Input: dimensioned drawing with shaded views. Units: mm. Origin: part minimum x, y, z. A direction names the side the tool comes from. Coordinates: 2 decimals unless noted, no trailing zeros. Loops run counter-clockwise (first coordinate to the right, second up) from the corner with the lowest first, then second, coordinate; pieces in that order, holes last.
Item 1: Line query: probe 1 along X at (y, z) = (4.75, 2.75); probe 2 along Z at (x, y) = (40, 4); probe 3 along X at (y, z) = (14.5, 25). Output: solid intervals per line, ascending.
Item 2: Section query D-D, the plane z = 27.75. Return the cut outline in (x, y), then the cut area to 3 significant figures.
Item 3: Reachability of the marked faces 1, 2 and 3 from +Z, -Z, +X, -X, +Y, -Y: full face, straight path, thin tool, end or side. Return the list, or none.
Item 4: Pull-direction query (Z, two-part tool) for the marked faces 4, 5, 6 and 7; classes: +Z half, -Z half, draft (parallel to the pull), parting line (faces both ways), or undercut.
Item 5: Section query B-B, the plane y = 10. Return the cut outline in (x, z), then the cut area to 3 significant figures.
Item 6: Section query A-A, the plane z = 8.75. Return the cut outline in (x, y).
Item 7: Pin query (flat end, axial travel): pin 1 Ø1.5 at (x, y) = (32.5, 3.5) entering from -Z; pin 2 Ø4.5 at (x, y) = (51, 4.5) entering from +Z; pin 3 Ø4.5 at (y, z) = (5.5, 27.5) entering from +X. Return the tip coordinate at first contact, or that it passes through.
Item 8: Section query C-C, the plane x = 11.5. Return the cut outline in (y, z), then the cut area to 3 significant figures.
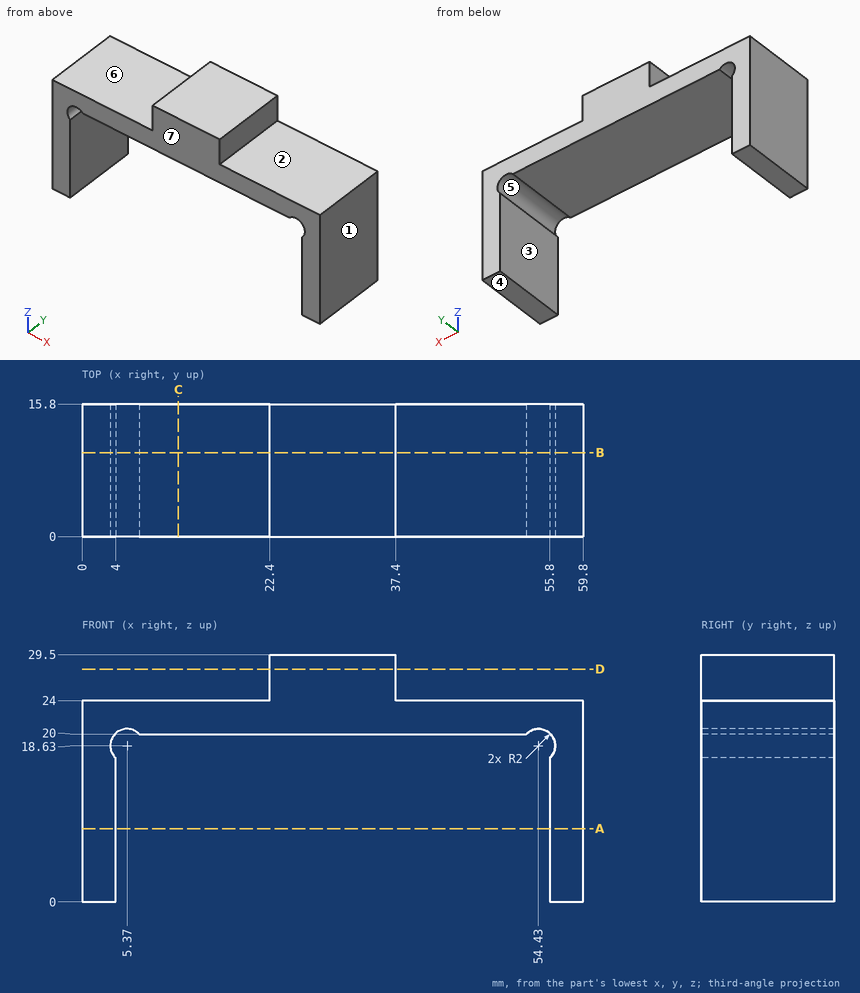
Verdict:
1. probe 1: x = 0 to 4, 55.8 to 59.8
1. probe 2: z = 20 to 24
1. probe 3: x = 22.4 to 37.4
2. outline: (22.4, 0) - (37.4, 0) - (37.4, 15.8) - (22.4, 15.8) - close
2. area: 237 mm2
3. face 1: +Z, -Z, +X, +Y, -Y
3. face 2: +Z, +X, +Y, -Y
3. face 3: -Z, +Y, -Y
4. face 4: -Z half
4. face 5: undercut
4. face 6: +Z half
4. face 7: draft
5. outline: (0, 0) - (4, 0) - (4, 17.17) arc R2 cw (long way) to (6.83, 20) - (52.97, 20) arc R2 cw (long way) to (55.8, 17.17) - (55.8, 0) - (59.8, 0) - (59.8, 24) - (37.4, 24) - (37.4, 29.5) - (22.4, 29.5) - (22.4, 24) - (0, 24) - close
5. area: 477 mm2
6. outline: (0, 0) - (4, 0) - (4, 15.8) - (0, 15.8) - close; (55.8, 0) - (59.8, 0) - (59.8, 15.8) - (55.8, 15.8) - close
7. pin 1: stops at z = 20
7. pin 2: stops at z = 24
7. pin 3: stops at x = 37.4
8. outline: (0, 20) - (15.8, 20) - (15.8, 24) - (0, 24) - close
8. area: 63.2 mm2
